Can you work these out from the model? Positions are in its coordinate system, mm. Face numbers are marked on the shaded views. A direction names the side the tool comes from. Give positions to 0.01 mm unless a question says otherwise; leave off trailing zeros. Order: outer loops, then holes, each group sorted by start corner. A loop starts at its lowest first (then second) coordinate and runs counter-clockwise, first axis right, second up. Notation, with made-up numbers: (-5, 77.5) - (41, 77.5) arc R8 cw to (41, 81.5) - close; hole circle Ø10 at (-18, 8.25). An arc over 180 degrees is marked (long way). Return JSON: item names as keys, results as strings.
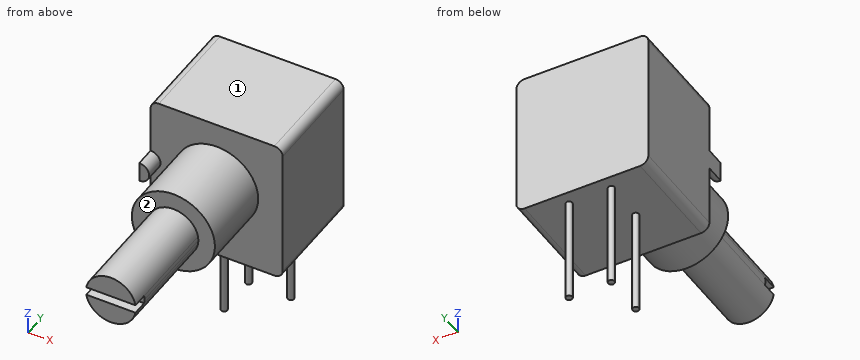
```python
from build123d import *

# Parameters (mm, degrees)
F0_R     = 5
F1_DEPTH = 12.7
F2_DEPTH = 22
F3_DEPTH = 20.2
F4_DEPTH = 9
F5_DEPTH = 2.36
F6_R     = 0.38
F7_DEPTH = 12.7


with BuildPart() as f1:
    # F0 (on Front) → F1 (new body)
    with BuildSketch(Plane.XZ):
        with BuildLine():
            Line((-6.94, -9.53), (6.94, -9.53))
            ThreePointArc((6.94, -9.53), (7.647107, -9.237107), (7.94, -8.53))
            Line((7.94, -8.53), (7.94, 6.92))
            ThreePointArc((7.94, 6.92), (7.647107, 7.627107), (6.94, 7.92))
            Line((6.94, 7.92), (-6.94, 7.92))
            ThreePointArc((-6.94, 7.92), (-7.647107, 7.627107), (-7.94, 6.92))
            Line((-7.94, 6.92), (-7.94, 1.19))
            ThreePointArc((-7.94, 1.19), (-6.75, 0), (-7.94, -1.19))
            Line((-7.94, -1.19), (-7.94, -8.53))
            ThreePointArc((-7.94, -8.53), (-7.647107, -9.237107), (-6.94, -9.53))
        make_face()
        Circle(F0_R, mode=Mode.SUBTRACT)
        Circle(F0_R)
        with BuildLine():
            ThreePointArc((2.95804, 0.5), (2.989492, 0.250879), (3, 0))
            ThreePointArc((3, 0), (2.989492, -0.250879), (2.95804, -0.5))
            ThreePointArc((2.95804, -0.5), (0, -3), (-2.95804, -0.5))
            ThreePointArc((-2.95804, -0.5), (-3, 0), (-2.95804, 0.5))
            ThreePointArc((-2.95804, 0.5), (0, 3), (2.95804, 0.5))
        make_face(mode=Mode.SUBTRACT)
        with BuildLine():
            Line((-7.94, 1.19), (-7.94, -1.19))
            ThreePointArc((-7.94, -1.19), (-6.75, 0), (-7.94, 1.19))
        make_face()
        with BuildLine():
            ThreePointArc((2.95804, -0.5), (2.989492, -0.250879), (3, 0))
            ThreePointArc((3, 0), (2.989492, 0.250879), (2.95804, 0.5))
            Line((2.95804, 0.5), (-2.95804, 0.5))
            ThreePointArc((-2.95804, 0.5), (-3, 0), (-2.95804, -0.5))
            Line((-2.95804, -0.5), (2.95804, -0.5))
        make_face()
        with BuildLine():
            Line((-2.95804, 0.5), (2.95804, 0.5))
            ThreePointArc((2.95804, 0.5), (0, 3), (-2.95804, 0.5))
        make_face()
        with BuildLine():
            ThreePointArc((-2.95804, -0.5), (0, -3), (2.95804, -0.5))
            Line((2.95804, -0.5), (-2.95804, -0.5))
        make_face()
    extrude(amount=-F1_DEPTH)

    # F0 (on Front) → F2 (join)
    with BuildSketch(Plane.XZ):
        with BuildLine():
            Line((-2.95804, 0.5), (2.95804, 0.5))
            ThreePointArc((2.95804, 0.5), (0, 3), (-2.95804, 0.5))
        make_face()
        with BuildLine():
            ThreePointArc((-2.95804, -0.5), (0, -3), (2.95804, -0.5))
            Line((2.95804, -0.5), (-2.95804, -0.5))
        make_face()
    extrude(amount=F2_DEPTH)

    # F0 (on Front) → F3 (join)
    with BuildSketch(Plane.XZ):
        with BuildLine():
            ThreePointArc((2.95804, -0.5), (2.989492, -0.250879), (3, 0))
            ThreePointArc((3, 0), (2.989492, 0.250879), (2.95804, 0.5))
            Line((2.95804, 0.5), (-2.95804, 0.5))
            ThreePointArc((-2.95804, 0.5), (-3, 0), (-2.95804, -0.5))
            Line((-2.95804, -0.5), (2.95804, -0.5))
        make_face()
    extrude(amount=F3_DEPTH)

    # F0 (on Front) → F4 (join)
    with BuildSketch(Plane.XZ):
        Circle(F0_R)
        with BuildLine():
            ThreePointArc((2.95804, 0.5), (2.989492, 0.250879), (3, 0))
            ThreePointArc((3, 0), (2.989492, -0.250879), (2.95804, -0.5))
            ThreePointArc((2.95804, -0.5), (0, -3), (-2.95804, -0.5))
            ThreePointArc((-2.95804, -0.5), (-3, 0), (-2.95804, 0.5))
            ThreePointArc((-2.95804, 0.5), (0, 3), (2.95804, 0.5))
        make_face(mode=Mode.SUBTRACT)
    extrude(amount=F4_DEPTH)

    # F0 (on Front) → F5 (join)
    with BuildSketch(Plane.XZ):
        with BuildLine():
            Line((-7.94, 1.19), (-7.94, -1.19))
            ThreePointArc((-7.94, -1.19), (-6.75, 0), (-7.94, 1.19))
        make_face()
    extrude(amount=F5_DEPTH)

    # F6 (on face) → F7 (join)
    with BuildSketch(Plane(origin=(0, 0, -9.53), x_dir=(1, 0, 0), z_dir=(0, 0, -1))):
        with Locations((-2.54, -5.97)):
            Circle(F6_R)
        with Locations((-2.54, -11.05)):
            Circle(F6_R)
        with Locations((2.54, -11.05)):
            Circle(F6_R)
    extrude(amount=F7_DEPTH)


solid = f1.part
```
1. If I drill on L1, parallel to Y at x = 4.75, z = -6.5; L2, parallel to Z at x = -6, y = 4; L3, parallel to Y at x = -2.25, z = -17.5, over which ranges is the centre line in solid material (lowest first)? Write a range as [from, to].
Checks:
{"L1": "[0, 12.7]", "L2": "[-9.53, 7.92]", "L3": "[5.72, 6.22], [10.8, 11.3]"}
2. Suppose I cut it at B-B (x = 0). List the corners of the cut face in (y, z) for me.
Checks:
{"outline": "(-22, -3) - (-9, -3) - (-9, -5) - (0, -5) - (0, -9.53) - (12.7, -9.53) - (12.7, 7.92) - (0, 7.92) - (0, 5) - (-9, 5) - (-9, 3) - (-22, 3) - (-22, 0.5) - (-20.2, 0.5) - (-20.2, -0.5) - (-22, -0.5) - close"}
3. Suppose I cut it at A-A (y = -0.5). List the corners of the cut face in (x, z) for me.
Checks:
{"outline": "(-7.94, -1.19) arc R1.19 ccw to (-7.94, 1.19) - close; circle Ø10 at (0, 0)"}
4. Suppose I cut it at D-D (z = -12). List the corners of the cut face in (x, y) for me, plus the area to 3 significant figures.
Checks:
{"outline": "circle Ø0.76 at (-2.54, 5.97); circle Ø0.76 at (-2.54, 11.05); circle Ø0.76 at (2.54, 11.05)", "area": "1.36 mm^2"}
5. For pin 1 Ø1.4 at (x, y) = (1.5, -21.5) entering from +Z; pin 2 Ø4 at (x, y) = (3, 6) entering from -Z; pin 3 Ø8 at (y, z) = (-16, 1.5) entering from -X, each with a flat end and sliding along its axis, tell me the tip position at first contact or that it passes through.
Checks:
{"pin 1": "z = 2.89", "pin 2": "z = -9.53", "pin 3": "x = -3"}
6. Suppose I cut it at C-C (y = 4.5). List the corners of the cut face in (x, z) for me.
Checks:
{"outline": "(-7.94, -8.53) arc R1 ccw to (-6.94, -9.53) - (6.94, -9.53) arc R1 ccw to (7.94, -8.53) - (7.94, 6.92) arc R1 ccw to (6.94, 7.92) - (-6.94, 7.92) arc R1 ccw to (-7.94, 6.92) - close"}
7. On a 3-axis mill with a long thin cutter (end or side, diameter ignored), from which of +Z, -Z, +X, -X, +Y, -Y can I reach the whole of each face in a straight line? I mean the marked faces 1 and 2. Say none if no direction works.
Checks:
{"face 1": "+Z, +X, -X, +Y, -Y", "face 2": "-Y"}
